```python
from build123d import *

# Parameters (mm, degrees)
F_1_4_0_2500_DOWEL_HOLE1_D = 6.35


with BuildPart() as part:
    # Sketch1 → Revolve1 (revolve)
    with BuildSketch(Plane.XY):
        Polygon((0, 4.064), (-15.3035, 4.064), (-15.3035, 19.05), (-14.2875, 19.05), (-14.2875, 15.875), (0, 15.875), align=None)
    revolve(axis=Axis((0, 0, 0), (-1, 0, 0)))

    # 1/4 (0.2500) Dowel Hole1 (through all)
    with Locations(Plane.ZY.offset(15.3035)):
        with Locations((0, 10.16), (8.798818102, -5.08), (-8.798818102, -5.08)):
            Hole(F_1_4_0_2500_DOWEL_HOLE1_D / 2)


solid = part.part
```
Here's how the part is built. I have some questions about the finished solid (model axes, mm). A direction names the side the tool comes from. Round coordinates to 2 decimals unless told otherwise and drop trailing zeros. Loops run counter-clockwise (first coordinate to the right, second up) from the corner with the lowest first, then second, coordinate; pieces in that order, holes last. Notation, with made-up numbers: (50, -14.75) -> (82, -14.75) arc R20 ccw to (82, 18.25) -> close; hole circle Ø6 at (70, -11). An arc over 180 degrees is marked (long way). Answer as CSV lines item,"result".
1. For pin 1 (2 mm diameter, centred on x = -8, y = -0.5, fed in from +Z) (3 decimals); pin 2 (4 mm diameter, centred on y = -5.08, z = -8.8, fed in from +X); pin 3 (1.5 mm diameter, centred on y = 14.5, z = -9.5, fed in from +X), each with a flat end and sliding along its axis, tell me the tip position at first contact or that it passes through.
Final values:
pin 1,"stops at z = 15.875"
pin 2,"passes through"
pin 3,"stops at x = -14.29"
2. Which directions (+Z, -Z, +X, -X, +Y, -Y) give clear straight access to the entire face, cutting with the end or side of a thin tool? Please do faces 1 (the face through (-7.54, -1.93, 9.21)), 2 (the face through (-7.044, -3.441, 15.497)).
Final values:
face 1,"+X, -X"
face 2,"+X"
3. If we section it at B-B on z = 7: Please give me the cut outline in (x, y), plus the area to 3 significant figures.
Final values:
outline,"(-15.3, -17.72) -> (-14.29, -17.72) -> (-14.29, -14.25) -> (0, -14.25) -> (0, -7.7) -> (-15.3, -7.7) -> close; (-15.3, -2.46) -> (0, -2.46) -> (0, 14.25) -> (-14.29, 14.25) -> (-14.29, 17.72) -> (-15.3, 17.72) -> close"
area,"363 mm^2"
4. Thinking about a two-plate mould opening in Z: for faces 3 (the face through (-14.79, -15.12, 11.59)), 4 (the face through (-7.759, -0.881, 3.967)), 5 (the face through (0, 3, 3)), which applies, released by +Z, released by -Z, zero draft, split by the parting line, or undercut?
Final values:
face 3,"split by the parting line"
face 4,"undercut"
face 5,"zero draft"
5. If we section it at A-A on z = 0: Count the separate pieces of the cut face and the enclosed holes in it, plus the area to 3 significant figures.
Final values:
separate pieces,"3"
enclosed holes,"0"
area,"271 mm^2"
6. If we section it at D-D on x = -8: Please give me the cut outline in (y, z) (3 decimals).
Final values:
outline,"circle Ø31.75 at (0, 0); hole circle Ø6.35 at (-5.08, -8.799); hole circle Ø6.35 at (-5.08, 8.799); hole circle Ø8.128 at (0, 0); hole circle Ø6.35 at (10.16, 0)"
7. If I drill on L1, parallel to Y at x = -9, z = 0 (3 decimals); L2, parallel to Z at x = -11, y = -3; L3, parallel to Z at x = -0.75, y = -3.5, over which ranges is the centre line in solid material (lowest first)?
Final values:
L1,"y = -15.875 to -4.064, 4.064 to 6.985, 13.335 to 15.875"
L2,"z = -15.59 to -11.2, -6.4 to -2.74, 2.74 to 6.4, 11.2 to 15.59"
L3,"z = -15.48 to -11.55, -6.04 to -2.07, 2.07 to 6.04, 11.55 to 15.48"
8. If we section it at C-C on y = 1: Please give me the cut outline in (x, z).
Final values:
outline,"(-15.3, -19.02) -> (-14.29, -19.02) -> (-14.29, -15.84) -> (0, -15.84) -> (0, -3.94) -> (-15.3, -3.94) -> close; (-15.3, 3.94) -> (0, 3.94) -> (0, 15.84) -> (-14.29, 15.84) -> (-14.29, 19.02) -> (-15.3, 19.02) -> close"
